Can you work these out from the model? Positions are in its coordinate system, mm. A direction names the side the tool comes from. Give positions to 0.01 mm unless a question says otherwise; leave off trailing zeros. Write each loop counter-clockwise with the first axis right and the second up, starting at its lowest first coordinate (ties: lowest second). Pieces come first, ordered by that corner, then holes.
Autodesk Inventor part; units mm, degrees
ref_plane "YZ Plane" through (0, 0, 0) normal (1, 0, 0) x (0, 1, 0)
ref_plane "XZ Plane" through (0, 0, 0) normal (0, 1, 0) x (-1, 0, 0)
ref_plane "XY Plane" through (0, 0, 0) normal (0, 0, 1) x (1, 0, 0)
sketch "Sketch1" plane through (0, 0, 0) normal (0, 0, 1) x (1, 0, 0)
  line L0 (0, 273.8452) -> (193.6378, 193.6378) construction
  line L1 (193.6378, 193.6378) -> (273.8452, 0) construction
  line L2 (273.8452, 0) -> (193.6378, -193.6378) construction
  line L3 (193.6378, -193.6378) -> (0, -273.8452) construction
  line L4 (0, -273.8452) -> (-193.6378, -193.6378) construction
  line L5 (-193.6378, -193.6378) -> (-273.8452, 0) construction
  line L6 (-273.8452, 0) -> (-193.6378, 193.6378) construction
  line L7 (-193.6378, 193.6378) -> (0, 273.8452)
  line L8 (-193.6378, 193.6378) -> (0, 273.8452)
  line L9 (-459.9272, 770.6562) -> (-219.7185, 870.1539)
  line L10 (-96.8189, 233.7415) -> (-339.8229, 820.405) construction
  line L11 (-219.7185, 870.1539) -> (0, 870.1539)
  line L12 (0, 870.1539) -> (0, 273.8452)
  line L13 (-459.9272, 770.6562) -> (-615.2917, 615.2917)
  line L14 (-615.2917, 615.2917) -> (-193.6378, 193.6378)
  point P0 (0, 0)
  point P1 (0, 0)
  dimension "d0" = 506
  dimension "d2" = 260
  dimension "d3" = 635
extrude "Extrusion1" add sketch "Sketch1" along normal mid plane 8
sketch "Sketch2" plane through (0, 0, 4) normal (0, 0, 1) x (1, 0, 0)
  line L0 (-219.7185, 870.1539) -> (-459.9272, 770.6562)
  line L1 (-459.9272, 770.6562) -> (-615.2917, 615.2917)
  line L2 (-235.0492, 528.2621) -> (-412.382, 454.8085)
  line L3 (-193.6378, 193.6378) -> (0, 273.8452)
  line L4 (-96.8189, 233.7415) -> (-339.8229, 820.405) construction
  line L5 (-615.2917, 615.2917) -> (-193.6378, 193.6378)
  line L6 (-412.382, 454.8085) -> (-572.8653, 615.2917)
  line L7 (-572.8653, 615.2917) -> (-442.9336, 745.2234)
  line L8 (-442.9336, 745.2234) -> (-342.2006, 786.9484)
  line L9 (-235.0492, 528.2621) -> (-342.2006, 786.9484)
  line L10 (-207.3328, 539.7426) -> (-30, 613.1963)
  line L11 (-30, 613.1963) -> (-30, 840.1539)
  line L12 (-30, 840.1539) -> (-213.7512, 840.1539)
  line L13 (-213.7512, 840.1539) -> (-314.4842, 798.4289)
  line L14 (-207.3328, 539.7426) -> (-314.4842, 798.4289)
  line L15 (0, 273.8452) -> (0, 870.1539)
  line L16 (-412.382, 454.8085) -> (-30, 613.1963) construction
  line L17 (-389.421, 431.8474) -> (-30, 580.7245)
  line L18 (-186.5988, 229.0252) -> (-30, 293.8906)
  line L19 (-30, 293.8906) -> (-30, 580.7245)
  line L20 (-186.5988, 229.0252) -> (-389.421, 431.8474)
  point P0 (0, 0)
  dimension "d11" = 30
  dimension "d12" = 280
  dimension "d13" = 30
  dimension "d14" = 30
  dimension "d15" = 15
  dimension "d21" = 30
  dimension "d22" = 30
  dimension "d23" = 30
  dimension "d24" = 30
extrude "Extrusion2" cut sketch "Sketch2" against normal up to surface (8 mm away)
fillet "Fillet1" radius 10 12 edges at (-572.8653, 615.2917, 0) (-342.2006, 786.9484, 0) (-235.0492, 528.2621, 0) (-412.382, 454.8085, 0) (-314.4842, 798.4289, 0) (-30, 840.1539, 0) (-30, 613.1963, 0) (-207.3328, 539.7426, 0) (-389.421, 431.8474, 0) (-30, 580.7245, 0) (-30, 293.8906, 0) (-186.5988, 229.0252, 0)
sketch "Sketch5" plane through (0, 0, 4) normal (0, 0, 1) x (1, 0, 0)
  line L0 (-219.7185, 870.1539) -> (-459.9272, 770.6562)
  line L1 (0, 870.1539) -> (-219.7185, 870.1539)
  line L2 (-459.9272, 770.6562) -> (-615.2917, 615.2917)
  line L3 (-615.2917, 615.2917) -> (-193.6378, 193.6378)
  line L4 (-193.6378, 193.6378) -> (0, 273.8452)
  line L5 (0, 273.8452) -> (0, 870.1539)
  line L6 (-15, 855.1539) -> (-216.7349, 855.1539) construction
  line L7 (-216.7349, 855.1539) -> (-451.4304, 757.9398) construction
  line L8 (-451.4304, 757.9398) -> (-594.0785, 615.2917) construction
  line L9 (-594.0785, 615.2917) -> (-190.1183, 211.3315) construction
  line L10 (-190.1183, 211.3315) -> (-15, 283.8679) construction
  line L11 (-15, 283.8679) -> (-15, 855.1539) construction
  line L12 (-375.5942, 437.5747) -> (-43.8268, 574.9973)
  line L13 (-211.1597, 548.9814) -> (-310.6574, 789.1901)
  line L14 (-415.9015, 437.1147) -> (-15, 603.1736) construction
  line L15 (-215.4508, 520.1442) -> (-334.0826, 806.5468) construction
  circle A0 centre (-334.0826, 806.5468) radius 2
  circle A1 centre (-215.4508, 520.1442) radius 2
  circle A2 centre (-294.54, 711.0824) radius 2
  circle A3 centre (-254.9973, 615.6179) radius 2
  circle A4 centre (-594.0785, 615.2917) radius 2
  circle A5 centre (-513.2865, 534.4997) radius 2
  circle A6 centre (-432.4944, 453.7076) radius 2
  circle A7 centre (-351.7024, 372.9156) radius 2
  circle A8 centre (-270.9103, 292.1235) radius 2
  circle A9 centre (-190.1183, 211.3315) radius 2
  circle A10 centre (-315.6917, 478.623) radius 2
  circle A11 centre (-102.5592, 247.5997) radius 2
  circle A12 centre (-516.2968, 693.0734) radius 2
  circle A13 centre (-435.7094, 764.4517) radius 2
  circle A14 centre (-15, 855.1539) radius 2
  circle A15 centre (-15, 740.8967) radius 2
  circle A16 centre (-15, 626.6395) radius 2
  circle A17 centre (-15, 512.3823) radius 2
  circle A18 centre (-15, 398.1251) radius 2
  circle A19 centre (-15, 283.8679) radius 2
  circle A20 centre (-115.2098, 561.6653) radius 2
  circle A21 centre (-125, 855.1539) radius 2
  circle A22 centre (-232.4559, 848.642) radius 2
  point P0 (0, 0)
  dimension "d32" = 15
  dimension "d33" = 15
  dimension "d34" = 15
  dimension "d35" = 4
  dimension "d37" = 103.33
  dimension "d38" = 103.33
  dimension "d43" = 114.2572
  dimension "d49" = 108.5
  dimension "d50" = 110
  dimension "d51" = 110
extrude "Extrusion4" cut sketch "Sketch5" against normal up to surface (8 mm away) contours A0 | A1 | A2 | A3 | A4 | A5 | A6 | A7 | A8 | A9 | A10 | A11 | A12 | A13 | A14 | A15 | A16 | A17 | A18 | A19 | A20 | A21 | A22
equation "\"d0\" = Барабан_габарит_по_кассетам"
equation "\"d2\" = Кассета_длина_грани"
equation "\"d3\" = Кассета_высота"
equation "\"d11\" = d13"
equation "\"d14\" = d13"
equation "\"d15\" = 0.5 * d13"
equation "\"d21\" = d13"
equation "\"d22\" = d13"
equation "\"d23\" = d13"
equation "\"d24\" = d13"
properties part number "ДМС 206 Крепление сетки к кассете"
1) Please list where these lines run through material, in increasing order: L1, parallel to Y at x = -235.5, z = -1.25; L2, parallel to Y at x = -94, z = 3; L3, parallel to X at y = 567, z = -0.5.
Values follow:
L1: y = 235.5 to 277.93, 495.6 to 607.74, 831.15 to 863.62
L2: y = 234.91 to 267.38, 554.21 to 586.69, 840.15 to 870.15
L3: x = -567 to -524.57, -251.09 to -218.62, -141.53 to -63.13, -30.08 to 0
2) Suppose I cut it at B-B on x = -392. Write out the boundary of the cut face in (y, z).
Values follow:
outline: (392, -4) - (463.25, -4) - (463.25, 4) - (392, 4) - close; (766.32, -4) - (798.79, -4) - (798.79, 4) - (766.32, 4) - close
3) Suppose I cut it at C-C on y = 583.5. Write out the boundary of the cut face in (x, z), plus the area to 3 significant figures.
Values follow:
outline: (-583.5, -4) - (-541.07, -4) - (-541.07, 4) - (-583.5, 4) - close; (-257.93, -4) - (-225.46, -4) - (-225.46, 4) - (-257.93, 4) - close; (-101.69, -4) - (0, -4) - (0, 4) - (-101.69, 4) - close
area: 1,410 mm2
4) Suppose I cut it at A-A on y = 350.5. Write out the boundary of the cut face in (x, z), plus the area to 3 significant figures.
Values follow:
outline: (-350.5, -4) - (-308.07, -4) - (-308.07, 4) - (-350.5, 4) - close; (-30, -4) - (0, -4) - (0, 4) - (-30, 4) - close
area: 579 mm2
5) For pin 1 Ø3 at (y, z) = (375, 3) entering from -X; pin 2 Ø3 at (x, y) = (-232.46, 848.64) entering from +Z; pin 3 Ø2.5 at (y, z) = (476, -1.5) entering from -X, each with a flat end and sliding along its axis, tell me the tip position at first contact or that it passes through.
Values follow:
pin 1: stops at x = -376.5
pin 2: passes through
pin 3: stops at x = -477.25
6) For faces 1 (the face through (-98.17, 233.18, -0.06)), 2 (the face through (-490.41, 532.836, 0.056)), which set-ups out of +Z, -Z, +X, -X, +Y, -Y let a thin tool reach every point of the face, with its end or its side?
Values follow:
face 1: +Z, -Z, +X, -Y
face 2: +Z, -Z
7) Suppose I cut it at D-D on z = 0. State how many separate pieces and enclosed holes the cut face has, plus the area to 3 significant figures.
Values follow:
separate pieces: 1
enclosed holes: 26
area: 80,100 mm2
8) If we mould it in two halves opening along Y, with no side actions, what happens to faces 3 (the face through (-341.5, 819.71, -0.06)), 4 (the face through (-283.768, 326.195, 0.056)), 5 (the face through (-241, 584, -4))? For each: +Y half, -Y half, draft (parallel to the pull), parting line (faces both ways), or undercut.
Values follow:
face 3: +Y half
face 4: undercut
face 5: draft
